Check sheet for the modelled part. Datum: model origin and axes. Units: mm. Round coordinates to 2 decimals unless told otherwise and drop trailing zeros. Order: outer loops, then holes, each group sorted by start corner. A loop starts at its lowest first (then second) coordinate and runs counter-clockwise, first axis right, second up. Notation, with made-up numbers: (-15, 49.25) -> (5, 49.25) arc R31 cw to (5, 74.25) -> close; hole circle Ø9 at (-10.75, -22). An arc over 180 degrees is marked (long way). Answer in a Markdown table with one row per item.
Autodesk Inventor part; units mm, degrees
ref_plane "YZ Plane" through (0, 0, 0) normal (1, 0, 0) x (0, 1, 0)
ref_plane "XZ Plane" through (0, 0, 0) normal (0, 1, 0) x (-1, 0, 0)
ref_plane "XY Plane" through (0, 0, 0) normal (0, 0, 1) x (1, 0, 0)
sketch "Skizze1" plane through (0, 0, 0) normal (0, 0, 1) x (1, 0, 0)
  line L0 (48, -48) -> (-48, -48)
  line L1 (-48, -48) -> (-48, 48)
  line L2 (-48, 48) -> (48, 48)
  line L3 (48, 48) -> (48, -48)
  line L4 (48, -48) -> (-48, 48) construction
  line L5 (-48, -48) -> (48, 48) construction
  circle A0 centre (0, 0) radius 32
  circle A1 centre (0, 0) radius 37 construction
  line L6 (-40, 40) -> (-48, 40)
  line L7 (-48, 40) -> (-48, 48)
  line L8 (-48, 48) -> (-40, 48)
  line L9 (-40, 48) -> (-40, 40)
  line L10 (-40, 40) -> (-48, 48) construction
  line L11 (-48, 40) -> (-40, 48) construction
  line L12 (-40, -40) -> (-48, -40)
  line L13 (-48, -40) -> (-48, -48)
  line L14 (-48, -48) -> (-40, -48)
  line L15 (-40, -48) -> (-40, -40)
  line L16 (-40, -40) -> (-48, -48) construction
  line L17 (-48, -40) -> (-40, -48) construction
  line L18 (40, -40) -> (48, -40)
  line L19 (48, -40) -> (48, -48)
  line L20 (48, -48) -> (40, -48)
  line L21 (40, -48) -> (40, -40)
  line L22 (40, -40) -> (48, -48) construction
  line L23 (48, -40) -> (40, -48) construction
  line L24 (40, 40) -> (48, 40)
  line L25 (48, 40) -> (48, 48)
  line L26 (48, 48) -> (40, 48)
  line L27 (40, 48) -> (40, 40)
  line L28 (40, 40) -> (48, 48) construction
  line L29 (48, 40) -> (40, 48) construction
  point P0 (-26.163, 26.163)
  point P1 (26.163, 26.163)
  point P2 (26.163, -26.163)
  point P3 (-26.163, -26.163)
  point P4 (-44, 44)
  point P5 (-44, -44)
  point P6 (44, -44)
  point P7 (44, 44)
  point P8 (-44, 44)
  point P9 (44, 44)
  point P10 (-44, -44)
  point P11 (44, -44)
  dimension "d0" = 96
  dimension "d1" = 96
  dimension "d41" = 64
  dimension "d42" = 74
  dimension "d43" = 8
  dimension "d44" = 8
extrude "Extrusion1" add sketch "Skizze1" along normal blind 3
hole "Bohrung2" at (-44, 44, 0) at (44, 44, 0) at (-44, -44, 0) at (44, -44, 0) direction (0, 0, 1) diameter 3.4 end through all
hole "Bohrung3" at (-26.163, 26.163, 0) at (26.163, 26.163, 0) at (26.163, -26.163, 0) at (-26.163, -26.163, 0) direction (0, 0, 1) diameter 4.2 end through all
equation "\"d0\" = d1"
properties part number "DayLightGlow_SpeakerBase"
Item 1: Scan lines: line 1 (Y direction, x = 44, z = 1.6); line 2 (Y direction, x = 0.5, z = 2.1). Record each from-to range of solid material in increasing order. Write a range as [from, to].
Result sheet:
| item | result |
|---|---|
| line 1 | y = [-48, -45.7], [-42.3, 42.3], [45.7, 48] |
| line 2 | y = [-48, -32], [32, 48] |
Item 2: Cross-section at B-B (y = 0). Record the boundary of the cut face in (x, z).
Result sheet:
| item | result |
|---|---|
| outline | (-48, 0) -> (-32, 0) -> (-32, 3) -> (-48, 3) -> close; (32, 0) -> (48, 0) -> (48, 3) -> (32, 3) -> close |
Item 3: Cross-section at A-A (x = -44). Record the boundary of the cut face in (y, z).
Result sheet:
| item | result |
|---|---|
| outline | (-48, 0) -> (-45.7, 0) -> (-45.7, 3) -> (-48, 3) -> close; (-42.3, 0) -> (42.3, 0) -> (42.3, 3) -> (-42.3, 3) -> close; (45.7, 0) -> (48, 0) -> (48, 3) -> (45.7, 3) -> close |
Item 4: Mould release check, pull along Y, two halves, no side actions. Record for faces 1 (the flat face through (48, 1, 1)), 2 (the cylindrical face through (-24.113, -26.618, 1.521)), 3 (the flat face through (-1, 48, 1)), 4 (the cylindrical face through (-42.97, -45.35, 1.52)): pulls with the +Y half, pulls with the -Y half, needs draft (parallel to the pull), parting line crosses it, or undercut.
Result sheet:
| item | result |
|---|---|
| face 1 | needs draft |
| face 2 | undercut |
| face 3 | pulls with the +Y half |
| face 4 | undercut |
Item 5: Depth check by flat-ended pin: P1, Ø3.5, axis at x = 26.163, y = 26.163, coming from the -Z side. Enter the tip coordinate at first touch or a pass-through.
Result sheet:
| item | result |
|---|---|
| P1 | passes through |
